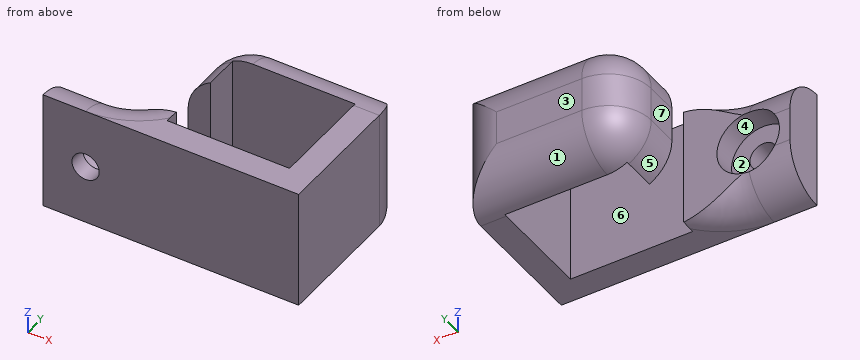
```python
from build123d import *

# Parameters (mm, degrees)
SKETCH1_W               = 30
SKETCH1_H               = 14
BOSS_EXTRUDE1_DEPTH     = 20
SKETCH2_W               = 10
SKETCH2_H               = 14.981059247
CUT_EXTRUDE1_DEPTH      = 20
FILLET1_R               = 5
SKETCH3_W               = 16.938954743
SKETCH3_H               = 3.286131709
CUT_EXTRUDE2_DEPTH      = 20
SKETCH4_W               = 7.5
SKETCH4_H               = 10.24752105
CUT_EXTRUDE3_DEPTH      = 20
CUT_EXTRUDE5_DEPTH      = 20
CUT_EXTRUDE5_DEPTH_BACK = 20
SKETCH5_R               = 1.6
CUT_EXTRUDE6_DEPTH      = 5
CUT_EXTRUDE6_DEPTH_BACK = 3
SKETCH6_R               = 3.75
SKETCH8_W               = 10.467205443
SKETCH8_H               = 5.426445144
CUT_EXTRUDE8_DEPTH      = 20
SKETCH9_W               = 2.170946208
SKETCH9_H               = 10.24752105
CUT_EXTRUDE9_DEPTH      = 20
SKETCH10_W              = 14.357250264
SKETCH10_H              = 12.211649431
CUT_EXTRUDE12_DEPTH     = 20


with BuildPart() as part:
    # Sketch1 → Boss-Extrude1 (new body)
    with BuildSketch(Plane(origin=(0, 0, 0), x_dir=(1, 0, 0), z_dir=(0, 1, 0))):
        with Locations((5.130024125, 0.849928215)):
            Rectangle(SKETCH1_W, SKETCH1_H)
    extrude(amount=BOSS_EXTRUDE1_DEPTH)

    # Sketch2 → Cut-Extrude1 (cut)
    with BuildSketch(Plane.XY.offset(6.150071785)):
        with Locations((-4.869975875, 12.509470377)):
            Rectangle(SKETCH2_W, SKETCH2_H)
    extrude(amount=-CUT_EXTRUDE1_DEPTH, mode=Mode.SUBTRACT)

    # Fillet1
    fillet1_edges = [part.edges().sort_by_distance(p)[0] for p in [
        (20.130024125, 20, -0.849928215),
        (10.130024125, 20, 6.150071785),
        (0.130024125, 20, -0.849928215),
        (-4.869975875, 5.018940753, -7.849928215),
        (10.130024125, 20, -7.849928215),
        (0.130024125, 5.018940753, -0.849928215),
        (0.130024125, 12.509470377, -7.849928215),
        (-4.869975875, 5.018940753, 6.150071785),
        (0.130024125, 12.509470377, 6.150071785),
    ]]
    fillet(fillet1_edges, radius=FILLET1_R)

    # Sketch3 → Cut-Extrude2 (cut)
    with BuildSketch(Plane(origin=(0, 0, -7.849928215), x_dir=(-1, 0, 0), z_dir=(0, 0, -1))):
        with Locations((-4.226478324, 9.498403921)):
            Rectangle(SKETCH3_W, SKETCH3_H)
    extrude(amount=-CUT_EXTRUDE2_DEPTH, mode=Mode.SUBTRACT)

    # Sketch4 → Cut-Extrude3 (cut)
    with BuildSketch(Plane(origin=(0, 0, -7.849928215), x_dir=(-1, 0, 0), z_dir=(0, 0, -1))):
        with Locations((-8.880024125, 9.876239475)):
            Rectangle(SKETCH4_W, SKETCH4_H)
    extrude(amount=-CUT_EXTRUDE3_DEPTH, mode=Mode.SUBTRACT)

    # Sketch5 → Cut-Extrude5 (cut, two sides: drawn at the far end of the back side and taken through both)
    with BuildSketch(Plane(origin=(0, 5.018940753, 0), x_dir=(1, 0, 0), z_dir=(0, 1, 0)).offset(-CUT_EXTRUDE5_DEPTH_BACK)):
        with Locations(Location((-4.869975875, 0.849928215, 0), (0, 0, 270))):
            Circle(SKETCH5_R)
    extrude(amount=CUT_EXTRUDE5_DEPTH + CUT_EXTRUDE5_DEPTH_BACK, mode=Mode.SUBTRACT)

    # Sketch6 → Cut-Extrude6 (cut, two sides: drawn at the far end of the back side and taken through both)
    with BuildSketch(Plane(origin=(0, 5.018940753, 0), x_dir=(1, 0, 0), z_dir=(0, 1, 0)).offset(-CUT_EXTRUDE6_DEPTH_BACK)):
        with Locations(Location((-4.869975875, 0.849928215, 0), (0, 0, 270))):
            Circle(SKETCH6_R)
    extrude(amount=CUT_EXTRUDE6_DEPTH + CUT_EXTRUDE6_DEPTH_BACK, mode=Mode.SUBTRACT)

    # Sketch8 → Cut-Extrude8 (cut)
    with BuildSketch(Plane(origin=(0, 0, -7.849928215), x_dir=(-1, 0, 0), z_dir=(0, 0, -1))):
        with Locations((0.103578597, 7.465701522)):
            Rectangle(SKETCH8_W, SKETCH8_H)
    extrude(amount=-CUT_EXTRUDE8_DEPTH, mode=Mode.SUBTRACT)

    # Sketch9 → Cut-Extrude9 (cut)
    with BuildSketch(Plane(origin=(0, 0, -7.849928215), x_dir=(-1, 0, 0), z_dir=(0, 0, -1))):
        with Locations((-13.715497229, 9.876239475)):
            Rectangle(SKETCH9_W, SKETCH9_H)
    extrude(amount=-CUT_EXTRUDE9_DEPTH, mode=Mode.SUBTRACT)

    # Sketch10 → Cut-Extrude12 (cut)
    with BuildSketch(Plane(origin=(0, 0, -7.849928215), x_dir=(-1, 0, 0), z_dir=(0, 0, -1))):
        with Locations((-9.948498564, 9.165448936)):
            Rectangle(SKETCH10_W, SKETCH10_H)
    extrude(amount=-CUT_EXTRUDE12_DEPTH, mode=Mode.SUBTRACT)


solid = part.part
```
Design review of the part built by this model. Coordinates are the model's own, in mm. Face numbers are marked on the shaded views. A direction names the side the tool comes from. Coordinates: 2 decimals unless noted, no trailing zeros. Order: outer loops, then holes, each group sorted by start corner. A loop starts at its lowest first (then second) coordinate and runs counter-clockwise, first axis right, second up. Notation, with made-up numbers: M 44,73 L 86,73 A18 cw 86,86 Z; hole C -17,57 d6. An arc over 180 degrees is marked long. Answer as a JSON object with one key per item and string values. Group by question number.
1) Add section C-C, the plane z = -1.25. Write out the cut boundary in (x, y), then the cut area to 3 significant figures.
2) Wall thickness on L1, parallel to Y at x = 6, z = 1.25; L2, parallel to Y at x = 4, z = -3.75; L3, parallel to X at y = 11, z = 0.75: over which ranges is each line inside the solid? List them lowest first.
3) For pin 1 (2 mm diameter, centred on y = 10.5, z = 4, fed in from -X); pin 2 (1.5 mm diameter, centred on y = 11, z = -0.5, fed in from -X); pin 3 (6 mm diameter, centred on x = -4.87, z = -0.85, fed in from -Y); pin 4 (5.5 mm diameter, centred on x = -0.5, z = -4, fed in from +Y), all flat-tipped, find the tip position at first contact; note any pin that passes through.
4) Tool access review of the marked faces 5, 6 and 7: name each direction out of +Z, -Z, +X, -X, +Y, -Y from which nothing blocks a thin tool from reaching the whole face with its end or side.
5) Add section D-D, the plane y = 17. Write out the cut boundary in (x, z).
6) Add section B-B, the plane y = 12.5. Write out the cut boundary in (x, z), then the cut area to 3 significant figures.
7) Add section A-A, the plane x = 12. Write out the cut boundary in (y, z), then the cut area to 3 significant figures.
8) Mouldability with a two-part tool opening along Z and no side actions: class the marked faces 1, 2, 3 and 4 as pulls with the +Z half, pulls with the -Z half, needs draft (parallel to the pull), parting line crosses it, or undercut.
Computed values:
{
 "1": {"outline": "M -9.87,0 L -6.42,0 L -6.42,2.02 L -8.6,2.02 L -8.6,5.02 L -9.87,5.02 Z; M -3.32,0 L 20.13,0 L 20.13,15 A5 ccw 15.13,20 L 5.13,20 A5 ccw 0.13,15 L 0.13,11.14 L 2.77,11.14 L 2.77,15.27 L 17.13,15.27 L 17.13,3.06 L 2.77,3.06 L 2.77,4.75 L -1.14,4.75 L -1.14,2.02 L -3.32,2.02 Z", "area": "218 mm^2"},
 "2": {"L1": "y = 0 to 3.06, 15.27 to 20", "L2": "y = 0 to 3.06, 15.27 to 19.79", "L3": "x = 17.13 to 20.13"},
 "3": {"pin 1": "stops at x = 0.58", "pin 2": "stops at x = 0.13", "pin 3": "stops at y = 0", "pin 4": "stops at y = 19"},
 "4": {"face 5": "-Z, -X, +Y", "face 6": "+Z, -Z", "face 7": "+Z, -Z, -X, +Y"},
 "5": {"outline": "M 0.55,-2.85 A4.58 ccw 5.13,-7.43 L 19.71,-7.43 L 19.71,5.73 L 5.13,5.73 A4.58 ccw 0.55,1.15 Z"},
 "6": {"outline": "M 0.13,-2.85 A5 ccw 2.77,-7.26 L 2.77,5.56 A5 ccw 0.13,1.15 Z; M 17.13,-7.85 L 20.13,-7.85 L 20.13,6.15 L 17.13,6.15 Z", "area": "69.2 mm^2"},
 "7": {"outline": "M 0,-7.85 L 3.06,-7.85 L 3.06,6.15 L 0,6.15 Z; M 15.27,-7.84 A5 ccw 20,-2.85 L 20,1.15 A5 ccw 15.27,6.14 Z", "area": "98.3 mm^2"},
 "8": {"face 1": "pulls with the -Z half", "face 2": "undercut", "face 3": "needs draft", "face 4": "undercut"}
}
